from build123d import *

# Parameters (mm, degrees)
BOSS_EXTRUDE1_DEPTH = 32.5
SKETCH2_W           = 55
SKETCH2_H           = 56.864750755
SKETCH2_H_2         = 60.635249245
CUT_EXTRUDE1_DEPTH  = 32.5
SKETCH4_R           = 8
BOSS_EXTRUDE2_DEPTH = 55
SKETCH5_W           = 38
SKETCH5_H           = 30
BOSS_EXTRUDE3_DEPTH = 20
SKETCH6_R           = 3
BOSS_EXTRUDE4_DEPTH = 3
FILLET1_R           = 2
FILLET3_R           = 2
FILLET5_R           = 5
FILLET6_R           = 5
FILLET7_R           = 5
FILLET8_R           = 5


with BuildPart() as part:
    # Sketch1 → Boss-Extrude1 (new body, symmetric)
    with BuildSketch(Plane(origin=(0, 0, 0), x_dir=(0, 0, -1), z_dir=(1, 0, 0))):
        with BuildLine():
            Line((1.875, -24.929588344), (101.3125, -17.450711841))
            ThreePointArc((101.3125, -17.450711841), (117.5, 0), (101.3125, 17.450711841))
            Line((101.3125, 17.450711841), (1.875, 24.929588344))
            ThreePointArc((1.875, 24.929588344), (-25, 0), (1.875, -24.929588344))
        make_face()
    extrude(amount=BOSS_EXTRUDE1_DEPTH, both=True)

    # Sketch2 → Cut-Extrude1 (cut, symmetric)
    with BuildSketch(Plane(origin=(0, 0, 0), x_dir=(1, 0, 0), z_dir=(0, 1, 0))):
        with Locations((0, 89.067624623)):
            Rectangle(SKETCH2_W, SKETCH2_H)
        with Locations((0, 5.317624623)):
            Rectangle(SKETCH2_W, SKETCH2_H_2)
    extrude(amount=CUT_EXTRUDE1_DEPTH, both=True, mode=Mode.SUBTRACT)

    # Sketch4 → Boss-Extrude2 (add)
    with BuildSketch(Plane(origin=(-27.5, 0, 0), x_dir=(0, 0, -1), z_dir=(1, 0, 0))):
        Circle(SKETCH4_R)
        with Locations((100, 0)):
            Circle(SKETCH4_R)
    extrude(amount=BOSS_EXTRUDE2_DEPTH)

    # Sketch5 → Boss-Extrude3 (add)
    with BuildSketch(Plane(origin=(32.5, 0, 0), x_dir=(0, 0, -1), z_dir=(1, 0, 0))):
        with Locations((16.635249245, 0)):
            Rectangle(SKETCH5_W, SKETCH5_H)
    extrude(amount=BOSS_EXTRUDE3_DEPTH)

    # Sketch6 → Boss-Extrude4 (add)
    with BuildSketch(Plane(origin=(0, 0, -35.635249245), x_dir=(-1, 0, 0), z_dir=(0, 0, -1))):
        with Locations((-42.5, 8)):
            Circle(SKETCH6_R)
        with Locations((-42.5, -8)):
            Circle(SKETCH6_R)
    extrude(amount=BOSS_EXTRUDE4_DEPTH)

    # Fillet1
    fillet1_edges = [part.edges().sort_by_distance(p)[0] for p in [
        (32.5, 0, -117.5),
        (32.5, 21.190150092, -51.59375),
        (32.5, 0, 25),
        (32.5, -21.190150092, -51.59375),
    ]]
    fillet(fillet1_edges, radius=FILLET1_R)

    # Fillet3
    fillet3_edges = [part.edges().sort_by_distance(p)[0] for p in [
        (-32.5, 21.190150092, -51.59375),
        (-32.5, 0, -117.5),
        (-32.5, -21.190150092, -51.59375),
        (-32.5, 0, 25),
    ]]
    fillet(fillet3_edges, radius=FILLET3_R)

    # Fillet5
    fillet5_edges = [part.edges().sort_by_distance(p)[0] for p in [
        (27.5, 0, -60.635249245),
    ]]
    fillet(fillet5_edges, radius=FILLET5_R)

    # Fillet6
    fillet6_edges = [part.edges().sort_by_distance(p)[0] for p in [
        (-27.5, 0, -60.635249245),
    ]]
    fillet(fillet6_edges, radius=FILLET6_R)

    # Fillet7
    fillet7_edges = [part.edges().sort_by_distance(p)[0] for p in [
        (-27.5, 0, -35.635249245),
    ]]
    fillet(fillet7_edges, radius=FILLET7_R)

    # Fillet8
    fillet8_edges = [part.edges().sort_by_distance(p)[0] for p in [
        (27.5, 0, -35.635249245),
    ]]
    fillet(fillet8_edges, radius=FILLET8_R)


solid = part.part
Could you check a few things on this model? Use its own coordinates, in mm. A direction names the side the tool comes from. Coordinates: 2 decimals unless noted, no trailing zeros. Order: outer loops, then holes, each group sorted by start corner. A loop starts at its lowest first (then second) coordinate and runs counter-clockwise, first axis right, second up. Notation, with made-up numbers: (61.25, 9) -> (105.25, 9) arc R22 ccw to (105.25, 44) -> close; hole circle Ø9 at (40.5, -12.75). An arc over 180 degrees is marked (long way). One line per question, with ' | ' between items.
Q1. Imagine slicing it at C-C on x = 42.5. Please give me the cut outline in (y, z), and give its area (3 significant figures).
Return value:
outline: (-15, -35.64) -> (-11, -35.64) -> (-11, -38.64) -> (-5, -38.64) -> (-5, -35.64) -> (5, -35.64) -> (5, -38.64) -> (11, -38.64) -> (11, -35.64) -> (15, -35.64) -> (15, 2.36) -> (-15, 2.36) -> close | area: 1,180 mm²
Q2. I'm going to push flat-ended pins straight in: P1, Ø5, axis at x = 42.5, y = -7.5, coming from the -Z side; P2, Ø22.5, axis at x = -6.5, y = -7.5, coming from the +Z side; P3, Ø6, axis at x = 27, z = -48.5, coming from the -Y side. Where does each tip first touch, or does it pass through?
Return value:
P1: z = -38.64 | P2: z = 8 | P3: y = -21.65
Q3. Imagine slicing it at A-A on x = 12.5. Please give me the cut outline in (y, z), and give its area (3 significant figures).
Return value:
outline: (-22.39, -35.64) -> (-20.51, -60.64) -> (20.51, -60.64) -> (22.39, -35.64) -> close; circle Ø16 at (0, -100); circle Ø16 at (0, 0) | area: 1,470 mm²
Q4. Thinking about a two-plate mould opening in X: for faces 4 (the face through (-31.93, -20.54, -52.24)), 5 (the face through (-27.5, 0, -9)), 6 (the face through (27.5, 0, -9)), 7 (the face through (29.021, -0.366, -117.496)), which applies, pulls with the +X half, pulls with the -X half, needs draft (parallel to the pull), parting line crosses it, or undercut?
Return value:
face 4: pulls with the -X half | face 5: undercut | face 6: undercut | face 7: needs draft
Q5. Imagine slicing it at B-B on y = 0. State how many separate pieces and enclosed holes the cut face has, and give its area (3 significant figures).
Return value:
separate pieces: 1 | enclosed holes: 2 | area: 5,340 mm²
Q6. On a 3-axis mill with a long thin cutter (end or side, diameter ignored), from which of +Z, -Z, +X, -X, +Y, -Y can I reach the whole of each face in a straight line? I mean faces 1 (the face through (42, -15, -16)), 2 (the face through (25.996, -0.319, -34.209)), 3 (the face through (43, -8, -38.635)). Say none if no direction works.
Return value:
face 1: +Z, -Z, +X, -Y | face 2: +Y, -Y | face 3: -Z, +X, +Y, -Y
Q7. If I drill on L1, parallel to X at y = 10.5, z = -89; L2, parallel to X at y = 9.5, z = -13.5; L3, parallel to Z at x = -23, y = 5 (3 decimals), over which ranges is the centre line in solid material (lowest first)?
Return value:
L1: -32.5 to -27.5, 27.5 to 32.5 | L2: -32.5 to -27.5, 27.5 to 52.5 | L3: -106.245 to -93.755, -60.66 to -35.61, -6.245 to 6.245
